Input: part model. Units: mm. Frame: model coordinates. A direction names the side the tool comes from. Coordinates: 2 decimals unless noted, no trailing zeros. Order: outer loops, then holes, each group sorted by start corner. A loop starts at its lowest first (then second) coordinate and runs counter-clockwise, first axis right, second up. Notation, with made-up numbers: (-11.5, 14.5) -> (-0.5, 14.5) arc R24 cw to (-0.5, 48.5) -> close; hole circle Ø10 at (-3, -39). An arc over 180 degrees is marked (long way). Use CSV: the item, a comma, the result in double quotes. Start each with the question number.
Autodesk Inventor part; units mm, degrees
ref_plane "YZ Plane" through (0, 0, 0) normal (1, 0, 0) x (0, 1, 0)
ref_plane "XZ Plane" through (0, 0, 0) normal (0, 1, 0) x (-1, 0, 0)
ref_plane "XY Plane" through (0, 0, 0) normal (0, 0, 1) x (1, 0, 0)
sketch "Sketch1" plane through (0, 0, 0) normal (0, 0, 1) x (1, 0, 0)
  circle A0 centre (-0.9432, 0.695) radius 7.9375
  circle A1 centre (-0.9432, 0.695) radius 4.7625
  dimension "d0" = 9.525
  dimension "d1" = 15.875
extrude "Extrusion1" add sketch "Sketch1" along normal blind 25.4
sketch "Sketch3" plane through (-0.9432, 0.695, 25.4) normal (0, 0, 1) x (1, 0, 0)
  circle A0 centre (0, 0) radius 7.9375
  circle A1 centre (0, 0) radius 7.9375
extrude "Extrusion2" add sketch "Sketch3" along normal blind 12.7
sketch "Sketch5" plane through (-0.9432, 0.695, 38.1) normal (0, 0, 1) x (1, 0, 0)
  circle A0 centre (0, 0) radius 7.9375
  line L0 (-1.5875, 1.5875) -> (1.5875, 1.5875)
  line L1 (1.5875, 1.5875) -> (1.5875, -1.5875)
  line L2 (1.5875, -1.5875) -> (-1.5875, -1.5875)
  line L3 (-1.5875, -1.5875) -> (-1.5875, 1.5875)
  point P0 (0, -1.5875)
  point P1 (1.5875, 0)
  dimension "d6" = 3.175
extrude "Extrusion3" cut sketch "Sketch5" against normal up to surface (12.7 mm away) contours L0 L1 L2 L3
properties part number "VEX Encoder shaft converter"
1. Section C-C on y = 4.25. Return loops of the section in (x, z), then the cut area to 3 significant figures.
2. Pull-direction query (X, two-part tool) for faces 1 (the face through (-8.873, 0.346, 18.783)), 2 (the face through (-2.531, 1, 32)), 3 (the face through (1, 1, 38.1)); classes: released by +X, released by -X, zero draft, split by the parting line, or undercut.
3. Section B-B on z = 33.5. Return loops of the section in (x, y) (1 decimal).
4. Material intervals for line 1 along Y through (x, z) = (2.25, 18.5); line 2 along Z through (x, y) = (-2, 3); line 3 along X through (y, z) = (-0.5, 13), sorted ascending.
5. Section A-A on y = 1.5. Return loops of the section in (x, z).
6. Access query for faces 4 (the face through (-1, -0.892, 32)), 5 (the face through (1, 1, 25.4)), 6 (the face through (-1.1, -4.5, 0)). Directions: +Z, -Z, +X, -X, +Y, -Y. A direction counts if a zero-diameter tool reaches every point of the face in a straight line with its end or side. Return the directions, or none.
7. Contact query for flat-ended pins moving along their axis: P1, Ø1, axis at y = 4, z = 13.5, coming from the -X side; P2, Ø3, axis at x = 1.5, y = 1, coming from the -Z side; P3, Ø3, axis at y = -1.5, z = 8, coming from the -X side. Output: stop coordinate, or through.
8. Section D-D on x = 3. Return loops of the section in (y, z), then the cut area to 3 significant figures.
Values follow:
1,outline,"(-8.04, 0) -> (-4.11, 0) -> (-4.11, 25.4) -> (2.23, 25.4) -> (2.23, 0) -> (6.15, 0) -> (6.15, 38.1) -> (-8.04, 38.1) -> close"
1,area,"380 mm2"
2,face 1,"split by the parting line"
2,face 2,"undercut"
2,face 3,"zero draft"
3,outline,"circle Ø15.9 at (-0.9, 0.7); hole (-2.5, -0.9) -> (0.6, -0.9) -> (0.6, 2.3) -> (-2.5, 2.3) -> close"
4,line 1,"y = -6.57 to -2.84, 4.23 to 7.96"
4,line 2,"z = 25.4 to 38.1"
4,line 3,"x = -8.79 to -5.55, 3.67 to 6.9"
5,outline,"(-8.84, 0) -> (-5.64, 0) -> (-5.64, 25.4) -> (-2.53, 25.4) -> (-2.53, 38.1) -> (-8.84, 38.1) -> close; (0.64, 25.4) -> (3.75, 25.4) -> (3.75, 0) -> (6.95, 0) -> (6.95, 38.1) -> (0.64, 38.1) -> close"
6,face 4,"+Z, -Z"
6,face 5,"-Z"
6,face 6,"-Z, +X, -X, +Y, -Y"
7,P1,"stops at x = -8.37"
7,P2,"stops at z = 25.4"
7,P3,"stops at x = -8.85"
8,outline,"(-6.19, 0) -> (-1.98, 0) -> (-1.98, 25.4) -> (3.37, 25.4) -> (3.37, 0) -> (7.58, 0) -> (7.58, 38.1) -> (-6.19, 38.1) -> close"
8,area,"389 mm2"
